The model under review builds one solid part; all positions refer to its coordinate system, in mm. A direction names the side the tool comes from. Give positions to 0.01 mm unless a question says otherwise; leave off trailing zeros. Loops run counter-clockwise (first coordinate to the right, second up) from the corner with the lowest first, then second, coordinate; pieces in that order, holes last. Notation, with made-up numbers: (52.25, 25) - (103.25, 25) arc R16 cw to (103.25, 36) - close; hole circle Ø6 at (13, 4). An arc over 180 degrees is marked (long way). Answer as a JSON object with one key per item and string values.
from build123d import *

# Parameters (mm, degrees)
SALIENTE_EXTRUIR1_DEPTH = 30
VACIADO1_T              = -1.5
CROQUIS4_W              = 36
CROQUIS4_H              = 8.3
CORTAR_EXTRUIR2_DEPTH   = 10
CROQUIS5_W              = 52.0366929
CROQUIS5_H              = 8.322917461
CORTAR_EXTRUIR3_DEPTH   = 10


with BuildPart() as part:
    # Croquis1 → Saliente-Extruir1 (new body)
    with BuildSketch(Plane(origin=(0, 0, 0), x_dir=(1, 0, 0), z_dir=(0, 1, 0))):
        Polygon((-28.5, -0.205897881), (-18, 19.794102119), (18, 19.794102119), (28.5, -0.205897881), align=None)
    extrude(amount=SALIENTE_EXTRUIR1_DEPTH)

    # Vaciado1
    vaciado1_openings = [part.faces().sort_by_distance(p)[0] for p in [
        (0, 0, -9.041413947),
    ]]
    offset(amount=VACIADO1_T, openings=vaciado1_openings, kind=Kind.INTERSECTION)

    # Croquis4 → Cortar-Extruir2 (cut)
    with BuildSketch(Plane(origin=(0, 0, -19.794102119), x_dir=(-1, 0, 0), z_dir=(0, 0, -1))):
        with Locations((0, 4.15)):
            Rectangle(CROQUIS4_W, CROQUIS4_H)
    extrude(amount=-CORTAR_EXTRUIR2_DEPTH, mode=Mode.SUBTRACT)

    # Croquis5 → Cortar-Extruir3 (cut)
    with BuildSketch(Plane(origin=(0, 0, -1.294102119), x_dir=(-1, 0, 0), z_dir=(0, 0, -1))):
        with Locations((0, 4.161458731)):
            Rectangle(CROQUIS5_W, CROQUIS5_H)
    extrude(amount=-CORTAR_EXTRUIR3_DEPTH, mode=Mode.SUBTRACT)


solid = part.part
Q1. Consider section B-B, the plane y = 6.25. State the section outline as (x, z) points, plus the area to 3 significant figures.
Results:
{"outline": "(-28.5, 0.21) - (-18, -19.79) - (-18, -16.57) - (-26.02, -1.29) - (-26.02, 0.21) - close; (18, -19.79) - (28.5, 0.21) - (26.02, 0.21) - (26.02, -1.29) - (18, -16.57) - close", "area": "63.5 mm^2"}
Q2. Clearance check with flat-ended pins moving along their axes: pin 1 Ø0.8 at (y, z) = (4.5, -0.5) entering from -X; pin 2 Ø10 at (y, z) = (13, -2.5) entering from -X; pin 3 Ø1.6 at (y, z) = (3.5, -17.5) entering from -X. State where each tip first meets the part, or that it passes through.
Results:
{"pin 1": "stops at x = -28.34", "pin 2": "stops at x = -28.5", "pin 3": "stops at x = -19.62"}
Q3. Consider section D-D, the plane z = -7. State the section outline as (x, y) points.
Results:
{"outline": "(-24.72, 0) - (-23.02, 0) - (-23.02, 28.5) - (23.02, 28.5) - (23.02, 0) - (24.72, 0) - (24.72, 30) - (-24.72, 30) - close"}
Q4. Consider section A-A, the plane y = 27.5. State the section outline as (x, z) points, plus the area to 3 significant figures.
Results:
{"outline": "(-28.5, 0.21) - (-18, -19.79) - (18, -19.79) - (28.5, 0.21) - close; hole (-26.02, -1.29) - (-17.09, -18.29) - (17.09, -18.29) - (26.02, -1.29) - close", "area": "197 mm^2"}
Q5. The part is to be moulded in two halves that separate along X. For faces 1 (the face through (23.18, 14.79, -9.93)), 2 (the face through (0, 8.3, -19)), 3 (the face through (18, 4, -18)), 4 (the face through (0, 21, 0.206)), say which applies: +X half, -X half, draft (parallel to the pull), parting line (faces both ways), or undercut.
Results:
{"face 1": "+X half", "face 2": "undercut", "face 3": "undercut", "face 4": "draft"}
Q6. Consider section C-C, the plane x = 5. State the section outline as (y, z) points, plus the area to 3 significant figures.
Results:
{"outline": "(8.3, -19.79) - (30, -19.79) - (30, 0.21) - (8.32, 0.21) - (8.32, -1.29) - (28.5, -1.29) - (28.5, -18.29) - (8.3, -18.29) - close", "area": "90.6 mm^2"}
Q7. To check wall thickness, follow probe 1 along Z at (x, y) = (-11.5, 10.25); probe 2 along Y at (x, z) = (-24, -1.75); probe 3 along X at (y, z) = (25, -15.25). State the ranges of each line that lie inside material, in increasing order. Write a range as [from, to].
Results:
{"probe 1": "z = [-19.79, -18.29], [-1.29, 0.21]", "probe 2": "y = [28.5, 30]", "probe 3": "x = [-20.39, -18.69], [18.69, 20.39]"}
Q8. For faces 5 (the face through (0, 18, -1.294)), 6 (the face through (26.018, 4, -1)), 7 (the face through (-18, 4, -18)), list the 3-axis set-ups (+Z, -Z, +X, -X, +Y, -Y) from which the entire face can be reached by the end or side of a thin tool; tool diameter is ignored.
Results:
{"face 5": "-Y", "face 6": "+Z, -Y", "face 7": "+Z, -Z, -Y"}
